from build123d import *

# Parameters (mm, degrees)
F0_W         = 63.5
F0_H         = 151
F1_DEPTH     = 2
F2_W         = 63.5
F2_H         = 1
F3_DEPTH     = 5
F4_W         = 5
F4_H         = 1.2
F5_DEPTH     = 10
F6_W         = 5
F6_H         = 1.2
F7_DEPTH     = 10
F8_W         = 4.3
F8_H         = 0.8
F9_DEPTH     = 9.75
F10_W        = 4.3
F10_H        = 0.8
F11_DEPTH    = 9.75
F12_W        = 2.75
F12_H        = 4.3
F13_DEPTH    = 1.2
F14_W        = 2.75
F14_H        = 4.3
F15_DEPTH    = 1.2
F16_W        = 2.75
F16_H        = 4.3
F17_DEPTH    = 1.2
F18_W        = 2.75
F18_H        = 4.3
F19_DEPTH    = 1.2
F20_W        = 2.75
F20_H        = 4.3
F21_DEPTH    = 1.2
F22_W        = 2.75
F22_H        = 4.3
F23_DEPTH    = 1.2
F28_W        = 3.25
F28_H        = 5
F29_W        = 3.25
F29_H        = 5
F27_W        = 3.25
F27_H        = 5
F26_W        = 3.25
F26_H        = 5
F25_W        = 3.25
F25_H        = 5
F24_W        = 3.25
F24_H        = 5
F30_DEPTH    = 5.801
F31_SIZE     = 1.6
F33_DEPTH    = 2.001
F34_T1_DEPTH = 2
F34_T3_DEPTH = 22
F35_R        = 8


# Not quite as in the source:
# - a fillet or chamfer that OpenCascade refuses, or shapes differently, is made with other operations: its cross-section is extruded or revolved along the edge and cut away or added


with BuildPart() as f1:
    # F0 (on Top) → F1 (new body)
    with BuildSketch(Plane.XY):
        with Locations((31.75, 75.5)):
            Rectangle(F0_W, F0_H)
    extrude(amount=F1_DEPTH)

    # F2 (on face) → F3 (join)
    with BuildSketch(Plane.XY.offset(2)):
        with Locations((31.75, 0.5)):
            Rectangle(F2_W, F2_H)
        with Locations((31.75, 150.5)):
            Rectangle(F2_W, F2_H)
    extrude(amount=F3_DEPTH)

    # F4 (on face) → F5 (cut)
    with BuildSketch(Plane.YZ.offset(63.5)):
        with Locations((13.5, 0.6)):
            Rectangle(F4_W, F4_H)
        with Locations((78, 0.6)):
            Rectangle(F4_W, F4_H)
        with Locations((142.5, 0.6)):
            Rectangle(F4_W, F4_H)
    extrude(amount=-F5_DEPTH, mode=Mode.SUBTRACT)

    # F6 (on face) → F7 (cut)
    with BuildSketch(Plane(origin=(0, 0, 0), x_dir=(0, -1, 0), z_dir=(-1, 0, 0))):
        with Locations((-137.5, 0.6)):
            Rectangle(F6_W, F6_H)
        with Locations((-73, 0.6)):
            Rectangle(F6_W, F6_H)
        with Locations((-8.5, 0.6)):
            Rectangle(F6_W, F6_H)
    extrude(amount=-F7_DEPTH, mode=Mode.SUBTRACT)

    # F8 (on face) → F9 (join)
    with BuildSketch(Plane.YZ.offset(63.5)):
        with Locations((137.5, 0.4)):
            Rectangle(F8_W, F8_H)
        with Locations((73, 0.4)):
            Rectangle(F8_W, F8_H)
        with Locations((8.5, 0.4)):
            Rectangle(F8_W, F8_H)
    extrude(amount=F9_DEPTH)

    # F10 (on face) → F11 (join)
    with BuildSketch(Plane(origin=(0, 0, 0), x_dir=(0, -1, 0), z_dir=(-1, 0, 0))):
        with Locations((-13.5, 0.4)):
            Rectangle(F10_W, F10_H)
        with Locations((-78, 0.4)):
            Rectangle(F10_W, F10_H)
        with Locations((-142.5, 0.4)):
            Rectangle(F10_W, F10_H)
    extrude(amount=F11_DEPTH)

    # F12 (on face) → F13 (join)
    with BuildSketch(Plane.XY.offset(0.8)):
        with Locations((71.875, 8.5)):
            Rectangle(F12_W, F12_H)
    extrude(amount=F13_DEPTH)

    # F14 (on face) → F15 (join)
    with BuildSketch(Plane.XY.offset(0.8)):
        with Locations((-8.375, 13.5)):
            Rectangle(F14_W, F14_H)
    extrude(amount=F15_DEPTH)

    # F16 (on face) → F17 (join)
    with BuildSketch(Plane.XY.offset(0.8)):
        with Locations((71.875, 73)):
            Rectangle(F16_W, F16_H)
    extrude(amount=F17_DEPTH)

    # F18 (on face) → F19 (join)
    with BuildSketch(Plane.XY.offset(0.8)):
        with Locations((-8.375, 78)):
            Rectangle(F18_W, F18_H)
    extrude(amount=F19_DEPTH)

    # F20 (on face) → F21 (join)
    with BuildSketch(Plane.XY.offset(0.8)):
        with Locations((71.875, 137.5)):
            Rectangle(F20_W, F20_H)
    extrude(amount=F21_DEPTH)

    # F22 (on face) → F23 (join)
    with BuildSketch(Plane.XY.offset(0.8)):
        with Locations((-8.375, 142.5)):
            Rectangle(F22_W, F22_H)
    extrude(amount=F23_DEPTH)

    # F28 (on face) + F29 (on face) + F27 (on face) + F26 (on face) + F25 (on face) + F24 (on face) → F30 (cut, through all)
    with BuildSketch(Plane(origin=(0, 0, 1.2), x_dir=(1, 0, 0), z_dir=(0, 0, -1))):
        with Locations((55.125, -13.5)):
            Rectangle(F28_W, F28_H)
    with BuildSketch(Plane(origin=(0, 0, 1.2), x_dir=(1, 0, 0), z_dir=(0, 0, -1))):
        with Locations((8.375, -8.5)):
            Rectangle(F29_W, F29_H)
    with BuildSketch(Plane(origin=(0, 0, 1.2), x_dir=(1, 0, 0), z_dir=(0, 0, -1))):
        with Locations((8.375, -73)):
            Rectangle(F27_W, F27_H)
    with BuildSketch(Plane(origin=(0, 0, 1.2), x_dir=(1, 0, 0), z_dir=(0, 0, -1))):
        with Locations((55.125, -78)):
            Rectangle(F26_W, F26_H)
    with BuildSketch(Plane(origin=(0, 0, 1.2), x_dir=(1, 0, 0), z_dir=(0, 0, -1))):
        with Locations((8.375, -137.5)):
            Rectangle(F25_W, F25_H)
    with BuildSketch(Plane(origin=(0, 0, 1.2), x_dir=(1, 0, 0), z_dir=(0, 0, -1))):
        with Locations((55.125, -142.5)):
            Rectangle(F24_W, F24_H)
    extrude(amount=-F30_DEPTH, mode=Mode.SUBTRACT)

    # F31
    f31_edges = [f1.edges().sort_by_distance(p)[0] for p in [
        (73.25, 8.5, 2),
        (73.25, 73, 2),
        (73.25, 137.5, 2),
        (-9.75, 142.5, 2),
        (-9.75, 78, 2),
        (-9.75, 13.5, 2),
    ]]
    chamfer(f31_edges, length=F31_SIZE)

    # F32 (on face) → F33 (cut, through all)
    with BuildSketch(Plane.XY.offset(2)):
        Polygon((7, 129), (7, 104.2), (56.5, 104.2), (56.5, 134), (47.5, 134), (47.5, 143), (16, 143), (16, 129), align=None)
        Polygon((7, 64.5), (7, 56.8), (56.5, 56.8), (56.5, 69.5), (47.5, 69.5), (47.5, 86.4947894041), (56.5, 86.4947894041), (56.5, 94.2), (7, 94.2), (7, 81.4947894041), (16, 81.4947894041), (16, 64.5), align=None)
        Polygon((7, 46.8), (7, 17), (16, 17), (16, 8), (47.5, 8), (47.5, 22), (56.5, 22), (56.5, 46.8), align=None)
    extrude(amount=-F33_DEPTH, mode=Mode.SUBTRACT)

    # F34: fillet of radius 4 on 22 edges, made by hand

    # F34_s2 → F34_t1 (join)
    with BuildSketch(Plane.XY):
        with BuildLine():
            ThreePointArc((20, 143), (17.1715728753, 141.8284271247), (16, 139))
            Line((16, 139), (16, 143))
            Line((16, 143), (20, 143))
        make_face()
        with BuildLine():
            ThreePointArc((7, 125), (8.1715728753, 127.8284271247), (11, 129))
            Line((11, 129), (7, 129))
            Line((7, 129), (7, 125))
        make_face()
        with BuildLine():
            ThreePointArc((7, 60.5), (8.1715728753, 63.3284271247), (11, 64.5))
            Line((11, 64.5), (7, 64.5))
            Line((7, 64.5), (7, 60.5))
        make_face()
        with BuildLine():
            ThreePointArc((52.5, 86.4947894041), (55.3284271247, 87.6663622794), (56.5, 90.4947894041))
            Line((56.5, 90.4947894041), (56.5, 86.4947894041))
            Line((56.5, 86.4947894041), (52.5, 86.4947894041))
        make_face()
        with BuildLine():
            ThreePointArc((52.5, 22), (55.3284271247, 23.1715728753), (56.5, 26))
            Line((56.5, 26), (56.5, 22))
            Line((56.5, 22), (52.5, 22))
        make_face()
        with BuildLine():
            ThreePointArc((43.5, 8), (46.3284271247, 9.1715728753), (47.5, 12))
            Line((47.5, 12), (47.5, 8))
            Line((47.5, 8), (43.5, 8))
        make_face()
        with BuildLine():
            ThreePointArc((56.5, 65.5), (55.3284271247, 68.3284271247), (52.5, 69.5))
            Line((52.5, 69.5), (56.5, 69.5))
            Line((56.5, 69.5), (56.5, 65.5))
        make_face()
        with BuildLine():
            ThreePointArc((56.5, 130), (55.3284271247, 132.8284271247), (52.5, 134))
            Line((52.5, 134), (56.5, 134))
            Line((56.5, 134), (56.5, 130))
        make_face()
        with BuildLine():
            ThreePointArc((47.5, 139), (46.3284271247, 141.8284271247), (43.5, 143))
            Line((43.5, 143), (47.5, 143))
            Line((47.5, 143), (47.5, 139))
        make_face()
        with BuildLine():
            ThreePointArc((7, 85.4947894041), (8.1715728753, 82.6663622794), (11, 81.4947894041))
            Line((11, 81.4947894041), (7, 81.4947894041))
            Line((7, 81.4947894041), (7, 85.4947894041))
        make_face()
        with BuildLine():
            ThreePointArc((7, 21), (8.1715728753, 18.1715728753), (11, 17))
            Line((11, 17), (7, 17))
            Line((7, 17), (7, 21))
        make_face()
        with BuildLine():
            ThreePointArc((7, 60.8), (8.1715728753, 57.9715728753), (11, 56.8))
            Line((11, 56.8), (7, 56.8))
            Line((7, 56.8), (7, 60.8))
        make_face()
        with BuildLine():
            ThreePointArc((56.5, 90.2), (55.3284271247, 93.0284271247), (52.5, 94.2))
            Line((52.5, 94.2), (56.5, 94.2))
            Line((56.5, 94.2), (56.5, 90.2))
        make_face()
        with BuildLine():
            ThreePointArc((16, 12), (17.1715728753, 9.1715728753), (20, 8))
            Line((20, 8), (16, 8))
            Line((16, 8), (16, 12))
        make_face()
    extrude(amount=F34_T1_DEPTH)

    # F34_s4 → F34_t3 (cut)
    with BuildSketch(Plane.XY.offset(-10)):
        with BuildLine():
            ThreePointArc((16, 133), (14.8284271247, 130.1715728753), (12, 129))
            Line((12, 129), (16, 129))
            Line((16, 129), (16, 133))
        make_face()
        with BuildLine():
            ThreePointArc((51.5, 134), (48.6715728753, 135.1715728753), (47.5, 138))
            Line((47.5, 138), (47.5, 134))
            Line((47.5, 134), (51.5, 134))
        make_face()
        with BuildLine():
            ThreePointArc((51.5, 69.5), (48.6715728753, 70.6715728753), (47.5, 73.5))
            Line((47.5, 73.5), (47.5, 69.5))
            Line((47.5, 69.5), (51.5, 69.5))
        make_face()
        with BuildLine():
            ThreePointArc((12, 81.4947894041), (14.8284271247, 80.3232165289), (16, 77.4947894041))
            Line((16, 77.4947894041), (16, 81.4947894041))
            Line((16, 81.4947894041), (12, 81.4947894041))
        make_face()
        with BuildLine():
            ThreePointArc((16, 68.5), (14.8284271247, 65.6715728753), (12, 64.5))
            Line((12, 64.5), (16, 64.5))
            Line((16, 64.5), (16, 68.5))
        make_face()
        with BuildLine():
            ThreePointArc((12, 17), (14.8284271247, 15.8284271247), (16, 13))
            Line((16, 13), (16, 17))
            Line((16, 17), (12, 17))
        make_face()
        with BuildLine():
            ThreePointArc((47.5, 82.4947894041), (48.6715728753, 85.3232165289), (51.5, 86.4947894041))
            Line((51.5, 86.4947894041), (47.5, 86.4947894041))
            Line((47.5, 86.4947894041), (47.5, 82.4947894041))
        make_face()
        with BuildLine():
            ThreePointArc((47.5, 18), (48.6715728753, 20.8284271247), (51.5, 22))
            Line((51.5, 22), (47.5, 22))
            Line((47.5, 22), (47.5, 18))
        make_face()
    extrude(amount=F34_T3_DEPTH, mode=Mode.SUBTRACT)

    # F35
    f35_edges = [f1.edges().sort_by_distance(p)[0] for p in [
        (7, 94.2, 1),
        (7, 46.8, 1),
        (56.5, 104.2, 1),
        (56.5, 56.8, 1),
        (7, 104.2, 1),
        (56.5, 46.8, 1),
    ]]
    fillet(f35_edges, radius=F35_R)


solid = f1.part
Geometry check sheet. Reference: the model listing, model coordinates, mm. A direction names the side the tool comes from. Give positions to 0.01 mm unless a question says otherwise; leave off trailing zeros. Order: outer loops, then holes, each group sorted by start corner. A loop starts at its lowest first (then second) coordinate and runs counter-clockwise, first axis right, second up.
1) Material ranges on probe 1 along Y at (x, z) = (22, 1.25); probe 2 along Y at (x, z) = (1, 4.25); probe 3 along X at (y, z) = (71, 1.5), recorded low to high.
Results are:
probe 1: y = 0 to 8, 46.8 to 56.8, 94.2 to 104.2, 143 to 151
probe 2: y = 0 to 1, 150 to 151
probe 3: x = 0 to 6.75, 10 to 16, 48.38 to 63.5, 70.5 to 72.15
2) Cross-section at B-B (z = 5.25). Record the boundary of the cut face in (x, y), then the cut area to 3 significant figures.
Results are:
outline: (0, 0) - (63.5, 0) - (63.5, 1) - (0, 1) - close; (0, 150) - (63.5, 150) - (63.5, 151) - (0, 151) - close
area: 127 mm2
3) Cross-section at D-D (x = 45). Record the boundary of the cut face in (y, z), then the cut area to 3 significant figures.
Results are:
outline: (0, 0) - (8.29, 0) - (8.29, 2) - (1, 2) - (1, 7) - (0, 7) - close; (46.8, 0) - (56.8, 0) - (56.8, 2) - (46.8, 2) - close; (94.2, 0) - (104.2, 0) - (104.2, 2) - (94.2, 2) - close; (142.71, 0) - (151, 0) - (151, 7) - (150, 7) - (150, 2) - (142.71, 2) - close
area: 83.2 mm2
4) Draft check along Y on faces 5 (the flat face through (0, 75.1, 1.4)), 6 (the cylindrical face through (17.141, 9.203, 0.986)), 7 (the flat face through (31, 0, 3)), 8 (the flat face through (67, 8, 0.8)). Enter one of: released by +Y, released by -Y, zero draft, split by the parting line, or undercut.
Results are:
face 5: undercut
face 6: undercut
face 7: released by -Y
face 8: zero draft
5) Tool access check on faces 1 (the flat face through (3, 73, 1.2)), 2 (the flat face through (31, 150, 4)), 3 (the cylindrical face through (8.14, 82.7, 0.99)), 4 (the flat face through (-3, 14, 0.8)). Record the directions out of +Z, -Z, +X, -X, +Y, -Y that give a thin tool (end or side, any length) a straight path to the whole face; none if there is none.
Results are:
face 1: -Z, -X
face 2: +Z, +X, -X
face 3: +Z, -Z
face 4: +Z, +Y, -Y
6) Cross-section at C-C (y = 19.5). Record the boundary of the cut face in (x, z).
Results are:
outline: (0, 0) - (7.29, 0) - (7.29, 2) - (0, 2) - close; (47.79, 0) - (63.5, 0) - (63.5, 2) - (47.79, 2) - close
7) Cross-section at A-A (x = 65). Record the boundary of the cut face in (y, z), then the cut area to 3 significant figures.
Results are:
outline: (6.35, 0) - (10.65, 0) - (10.65, 0.8) - (6.35, 0.8) - close; (70.85, 0) - (75.15, 0) - (75.15, 0.8) - (70.85, 0.8) - close; (135.35, 0) - (139.65, 0) - (139.65, 0.8) - (135.35, 0.8) - close
area: 10.3 mm2
8) Gauge pin test, flat ends, axial feed: pin 1 (1.5 mm diameter, centred on x = 59, y = 143, fed in from -Z); pin 2 (5 mm diameter, centred on x = 26, y = 56.5, fed in from -Z); pin 3 (1.3 mm diameter, centred on y = 78, z = 1, fed in from +X); pin 4 (0.9 mm diameter, centred on x = 71.5, y = 137, fed in from +Z). Record the tip position at first contact, or that the pin passes through.
Results are:
pin 1: stops at z = 1.2
pin 2: stops at z = 0
pin 3: stops at x = 63.5
pin 4: stops at z = 2
